The listing builds one solid part. Answer for the finished solid, in the listing's coordinates (mm). A direction names the side the tool comes from. Coordinates: 2 decimals unless noted, no trailing zeros. Write each loop counter-clockwise with the first axis right and the second up, starting at its lowest first coordinate (ties: lowest second). Pieces come first, ordered by that corner, then holes.
from build123d import *

# Parameters (mm, degrees)
F0_W                 = 20
F0_H                 = 20
F1_DEPTH             = 20
F5_D                 = 5
F5_CBORE_D           = 10
F5_CBORE_DEPTH       = 15
F5_ON_F3_D           = 5
F5_ON_F3_CBORE_D     = 10
F5_ON_F3_CBORE_DEPTH = 15
F5_ON_F4_D           = 5
F5_ON_F4_CBORE_D     = 10
F5_ON_F4_CBORE_DEPTH = 15


with BuildPart() as f1:
    # F0 (on Top) → F1 (new body)
    with BuildSketch(Plane.XY):
        Rectangle(F0_W, F0_H)
    extrude(amount=F1_DEPTH)

    # F5 (through all)
    with Locations(Plane.XZ.offset(10)):
        with Locations((0, 10)):
            CounterBoreHole(F5_D / 2, F5_CBORE_D / 2, F5_CBORE_DEPTH)

    # F5 on F3 (through all)
    with Locations(Plane.YZ.offset(10)):
        with Locations((0, 10)):
            CounterBoreHole(F5_ON_F3_D / 2, F5_ON_F3_CBORE_D / 2, F5_ON_F3_CBORE_DEPTH)

    # F5 on F4 (through all)
    with Locations(Plane.XY.offset(20)):
        with Locations((0, 0)):
            CounterBoreHole(F5_ON_F4_D / 2, F5_ON_F4_CBORE_D / 2, F5_ON_F4_CBORE_DEPTH)


solid = f1.part
Q1. Determine the mould class of faces 1 (the face through (-2, -2, 0)), 2 (the face through (2, 5, 8)), 3 (the face through (0.54, -2.44, 2.46)) for opening direction Y: released by +Y, released by -Y, zero draft, split by the parting line, or undercut.
Answers below:
face 1: zero draft
face 2: released by -Y
face 3: undercut
Q2. The part is cut by section B-B, the plane y = -4. Write down the section's boundary in (x, z), then the cut area to 3 significant figures.
Answers below:
outline: (-10, 0) - (10, 0) - (10, 7) - (4, 7) arc R5 cw to (3, 6) - (3, 5) - (-3, 5) - (-3, 6) arc R5 cw to (-4, 7) - (-5, 7) - (-5, 13) - (-4, 13) arc R5 cw to (-3, 14) - (-3, 20) - (-10, 20) - close; (3, 14) arc R5 cw to (4, 13) - (10, 13) - (10, 20) - (3, 20) - close
area: 254 mm2
Q3. The part is cut by section C-C, the plane y = -1. Write down the section's boundary in (x, z), then the cut area to 3 significant figures.
Answers below:
outline: (-10, 0) - (-2.29, 0) - (-2.29, 5) - (-4.9, 5) - (-4.9, 5.1) - (-5, 5.1) - (-5, 7.71) - (-10, 7.71) - close; (-10, 12.29) - (-5, 12.29) - (-5, 14.9) - (-4.9, 14.9) - (-4.9, 20) - (-10, 20) - close; (2.29, 0) - (10, 0) - (10, 5.1) - (4.9, 5.1) - (4.9, 5) - (2.29, 5) - close; (4.9, 14.9) - (10, 14.9) - (10, 20) - (4.9, 20) - close
area: 156 mm2
Q4. Find the intervals of material crossed by probe 1 along X at (y, z) = (7.85, 10); probe 2 along Y at (x, z) = (0, 18.25), in increasing order.
Answers below:
probe 1: x = -10 to -2.5, 2.5 to 10
probe 2: y = -10 to -5, 5 to 10
Q5. The part is cut by section D-D, the plane z = 3.5. Write down the section's boundary in (x, y).
Answers below:
outline: (-10, -10) - (10, -10) - (10, 10) - (-10, 10) - close; hole circle Ø5 at (0, 0)
Q6. The part is cut by section A-A, the plane z = 7. Write down the section's boundary in (x, y).
Answers below:
outline: (-10, -10) - (-4, -10) - (-4, -4) - (-5, -4) - (-5, 4) - (-4, 4) - (-4, 5) - (4, 5) - (4, 4) - (10, 4) - (10, 10) - (-10, 10) - close; (4, -10) - (10, -10) - (10, -4) - (4, -4) - close
Q7. Given pin 1 (6 mm diameter, centred on x = 0, z = 10, fed in from -Y); pin 2 (6.5 mm diameter, centred on x = 0, y = 0, fed in from +Z); pin 3 (8 mm diameter, centred on x = 1, z = 10.5, fed in from -Y), each flat-ended and moving along its own axis, determine where each tip first touches the part or whether it passes through.
Answers below:
pin 1: stops at y = 5
pin 2: stops at z = 5
pin 3: stops at y = -10
Q8. Which of the six approach directions +Z, -Z, +X, -X, +Y, -Y give full straight-line access (tool end or side, diameter ignored) to faces 4 (the face through (10, -2, 5)), 5 (the face through (-4.54, -3.55, 6.48)), 6 (the face through (-3.52, 4.54, 13.55)), 7 (the face through (-3.55, -3.52, 5.46))?
Answers below:
face 4: +Z, -Z, +X, +Y, -Y
face 5: +X
face 6: -Y
face 7: +Z
